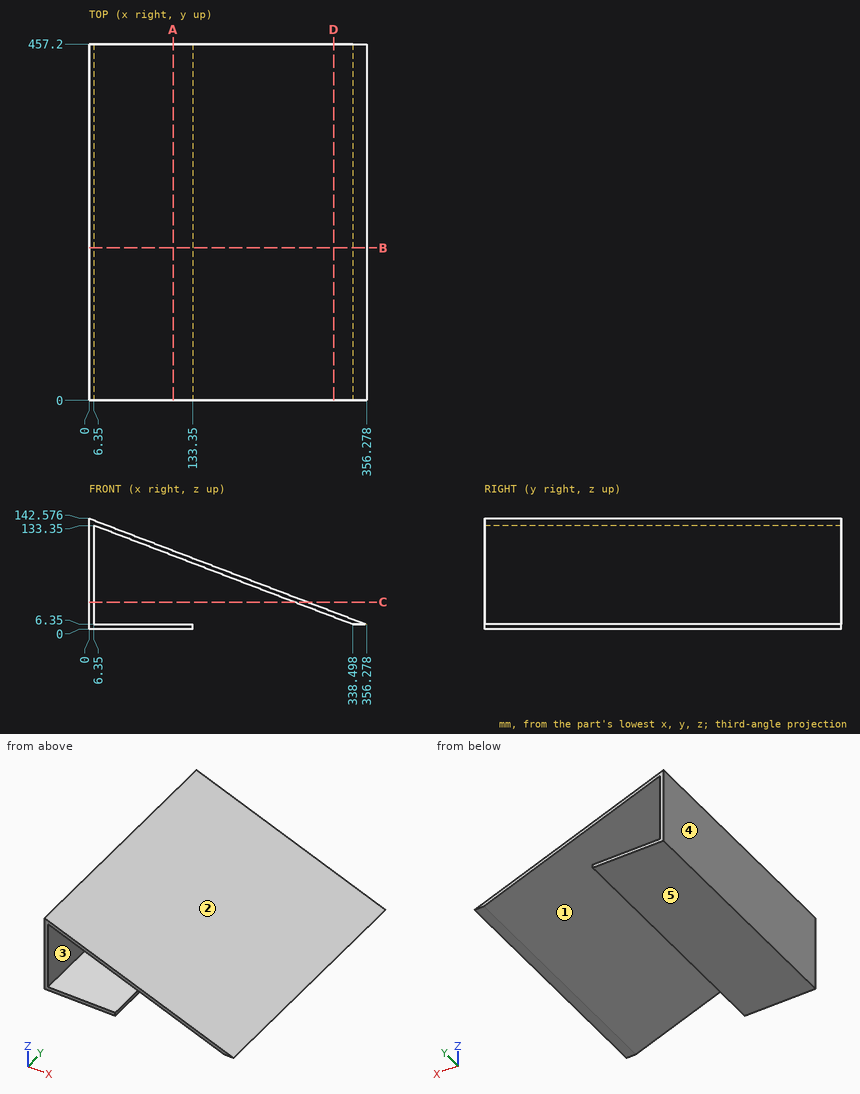
For this review, use the dimensioned drawing (mm, ordinates from the lowest corner) and the shaded views. A direction names the side the tool comes from. Coordinates: 2 decimals unless noted, no trailing zeros. Order: outer loops, then holes, each group sorted by start corner. A loop starts at its lowest first (then second) coordinate and runs counter-clockwise, first axis right, second up. Notation, with made-up numbers: M -33.75,70.5 L 13.25,70.5 A23 ccw 13.25,86.5 Z; hole C 30.5,67 d9. An arc over 180 degrees is marked long. Answer as a JSON object with one key per item and string values. Group by question number.
1) Mouldability with a two-part tool opening along X and no side actions: class the marked faces 3, 4 and 5 as pulls with the +X half, pulls with the -X half, needs draft (parallel to the pull), parting line crosses it, or undercut.
2) Add section A-A, the plane x = 108. Write out the cut boundary in (y, z).
3) Add section C-C, the plane z = 35. Write out the cut boundary in (x, y), then the cut area to 3 significant figures.
4) Tool access review of the marked faces 1 and 2: name each direction out of +Z, -Z, +X, -X, +Y, -Y from which nothing blocks a thin tool from reaching the whole face with its end or side.
5) Add section D-D, the plane x = 314. Write out the cut boundary in (y, z) (1 decimal), then the cut area to 3 significant figures.
6) For pin 1 (19.5 mm diameter, centred on x = 351.5, y = 132, fed in from -Z); pin 2 (3 mm diameter, centred on x = 287.5, y = 409, fed in from +Z); pin 3 (5 mm diameter, centred on y = 257, z = 3, fed in from +X), all flat-tipped, find the tip position at first contact; note any pin that passes through.
7) Wall thickness on L1, parallel to Z at x = 23, y = 387; L2, parallel to Z at x = 33, y = 93.5; L3, parallel to Z at x = 313.5, y = 438: over which ranges is each line inside the solid? List them lowest first.
8) Add section B-B, the plane y = 195.5. Write out the cut boundary in (x, z), then the cut area to 3 significant figures.
Computed values:
{
 "1": {"face 3": "undercut", "face 4": "pulls with the -X half", "face 5": "needs draft"},
 "2": {"outline": "M 0,0 L 457.2,0 L 457.2,6.35 L 0,6.35 Z; M 0,94.48 L 457.2,94.48 L 457.2,101.28 L 0,101.28 Z"},
 "3": {"outline": "M 0,0 L 6.35,0 L 6.35,457.2 L 0,457.2 Z; M 263.57,0 L 281.35,0 L 281.35,457.2 L 263.57,457.2 Z", "area": "11,000 mm^2"},
 "4": {"face 1": "+Y, -Y", "face 2": "+Z, +X, +Y, -Y"},
 "5": {"outline": "M 0,15.7 L 457.2,15.7 L 457.2,22.5 L 0,22.5 Z", "area": "3,110 mm^2"},
 "6": {"pin 1": "stops at z = 6.35", "pin 2": "stops at z = 33.22", "pin 3": "stops at x = 133.35"},
 "7": {"L1": "z = 0 to 6.35, 126.98 to 133.78", "L2": "z = 0 to 6.35, 123.16 to 129.96", "L3": "z = 15.91 to 22.71"},
 "8": {"outline": "M 0,0 L 133.35,0 L 133.35,6.35 L 6.35,6.35 L 6.35,133.35 L 338.5,6.35 L 356.28,6.35 L 0,142.58 Z", "area": "4,020 mm^2"}
}
